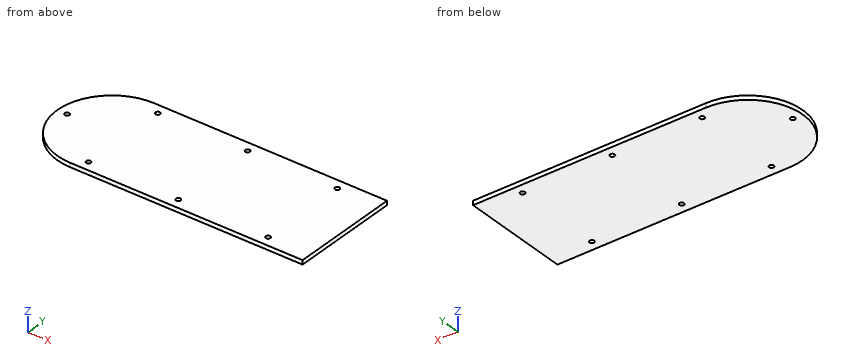
```python
from build123d import *

# Parameters (mm, degrees)
SKETCH_R  = 1.65
PAD_DEPTH = 3


with BuildPart() as part:
    # Sketch → Pad (new body)
    with BuildSketch(Plane.XY):
        with BuildLine():
            ThreePointArc((0, 39), (-39, 0), (0, -39))
            Line((166, -39), (0, -39))
            Line((166, 39), (166, -39))
            Line((0, 39), (166, 39))
        make_face()
        with Locations((-32, 0)):
            Circle(SKETCH_R, mode=Mode.SUBTRACT)
        with Locations((8, 32)):
            Circle(SKETCH_R, mode=Mode.SUBTRACT)
        with Locations((72, 32)):
            Circle(SKETCH_R, mode=Mode.SUBTRACT)
        with Locations((136, 32)):
            Circle(SKETCH_R, mode=Mode.SUBTRACT)
        with Locations((8, -32)):
            Circle(SKETCH_R, mode=Mode.SUBTRACT)
        with Locations((72, -32)):
            Circle(SKETCH_R, mode=Mode.SUBTRACT)
        with Locations((136, -32)):
            Circle(SKETCH_R, mode=Mode.SUBTRACT)
    extrude(amount=PAD_DEPTH)


solid = part.part
```
Work out the finished part from the listing and answer in its coordinate system (mm). Round coordinates to 2 decimals unless told otherwise and drop trailing zeros. Write each loop counter-clockwise with the first axis right and the second up, starting at its lowest first coordinate (ties: lowest second). Pieces come first, ordered by that corner, then holes. Notation, with made-up numbers: (30, 77) - (50, 77) arc R19 cw to (50, 97) - close; hole circle Ø9 at (25, 44). An arc over 180 degrees is marked (long way). Return JSON: item names as keys, results as strings. Group by question number.
Q1. The part is cut by section C-C on y = -18.5. Write down the section's boundary in (x, z).
Q2. This flat-tipped pin is pushed along its axis until it touches: pin 1 Ø2 at (x, y) = (72, -32) entering from -Z. Where does it stop, or does it pass through?
Q3. Find the intervals of material crossed by L1, parallel to Y at x = 8, z = 0.8; L2, parallel to Y at x = -32, z = 0.9; L3, parallel to X at y = 5, z = 2.65, in increasing order.
Q4. The part is cut by section B-B on x = -21. Write down the section's boundary in (y, z).
Q5. The part is cut by section A-A on z = 2.45. Write down the section's boundary in (x, y), then the cut area to 3 significant figures.
Solved:
{
 "1": {"outline": "(-34.33, 0) - (166, 0) - (166, 3) - (-34.33, 3) - close"},
 "2": {"pin 1": "through"},
 "3": {"L1": "-39 to -33.65, -30.35 to 30.35, 33.65 to 39", "L2": "-22.29 to -1.65, 1.65 to 22.29", "L3": "-38.68 to 166"},
 "4": {"outline": "(-32.86, 0) - (32.86, 0) - (32.86, 3) - (-32.86, 3) - close"},
 "5": {"outline": "(0, -39) - (166, -39) - (166, 39) - (0, 39) arc R39 ccw to start; hole circle Ø3.3 at (-32, 0); hole circle Ø3.3 at (8, -32); hole circle Ø3.3 at (8, 32); hole circle Ø3.3 at (72, -32); hole circle Ø3.3 at (72, 32); hole circle Ø3.3 at (136, -32); hole circle Ø3.3 at (136, 32)", "area": "15,300 mm²"}
}
